Could you check a few things on this model? Use its own coordinates, in mm. Give positions to 0.01 mm unless a question says otherwise; leave off trailing zeros. Loops run counter-clockwise (first coordinate to the right, second up) from the corner with the lowest first, then second, coordinate; pieces in that order, holes last. Notation, with made-up numbers: M 34.5,79 L 82.5,79 A25 ccw 82.5,100 Z; hole C 38,-27.5 d10. An arc over 180 degrees is marked long. Return JSON: item names as keys, results as strings. Group by question number.
1. Please list where these lines run through material, in increasing order: line 1 (X direction, y = 13, z = -125); line 2 (Z direction, x = 20, y = 13); line 3 (X direction, y = 13.5, z = -129.5).
2. If we section it at B-B (y = 34.5): Write out the boundary of the cut face in (x, z), plus the area to 3 significant figures.
3. For pin 1 (0.5 mm diameter, centred on x = 0, z = 69.5, fed in from +Y); pin 2 (7 mm diameter, centred on x = -20.5, z = -127.5, fed in from +Y); pin 3 (4.5 mm diameter, centred on x = -19, z = -123, fed in from +Y), each with a flat end and sliding along its axis, tell me the tip position at first contact or that it passes through.
4. If we section it at C-C (x = 20.5): Write out the boundary of the cut face in (y, z).
5. If we section it at A-A (z = -125): Write out the boundary of the cut face in (x, y), plus the area to 3 significant figures.
6. If we section it at D-D (z = -32.5): Write out the boundary of the cut face in (x, y), plus the area to 3 significant figures.
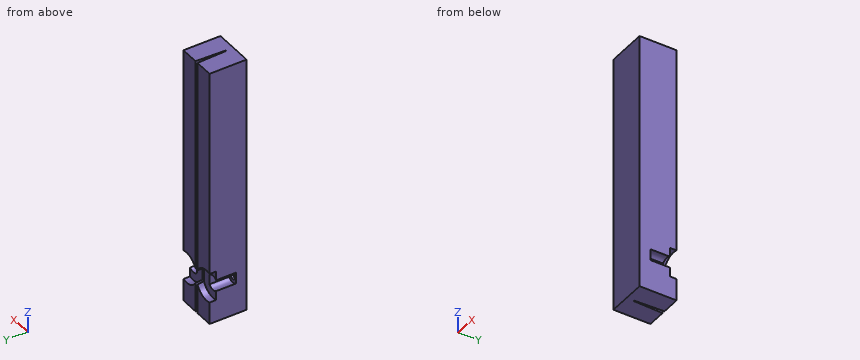
```python
from build123d import *

# Parameters (mm, degrees)
SKETCH1_W           = 54
SKETCH1_H           = 350
BOSS_EXTRUDE1_DEPTH = 50
CUT_EXTRUDE2_DEPTH  = 355.582853505
SKETCH7_R           = 21
SKETCH7_R_2         = 10
CUT_EXTRUDE4_DEPTH  = 9
CUT_EXTRUDE5_DEPTH  = 35.5
CUT_EXTRUDE6_DEPTH  = 3
CUT_EXTRUDE7_DEPTH  = 9


with BuildPart() as part:
    # Sketch1 → Boss-Extrude1 (new body)
    with BuildSketch(Plane(origin=(0, 0, 0), x_dir=(1, 0, 0), z_dir=(0, 1, 0))):
        Rectangle(SKETCH1_W, SKETCH1_H)
    extrude(amount=BOSS_EXTRUDE1_DEPTH)

    # Sketch3 → Cut-Extrude2 (cut, through all)
    with BuildSketch(Plane.XY.offset(175)):
        Polygon((-0.5, 10), (-2, 50), (2, 50), (0.5, 10), align=None)
    extrude(amount=-CUT_EXTRUDE2_DEPTH, mode=Mode.SUBTRACT)

    # Sketch7 → Cut-Extrude4 (cut)
    with BuildSketch(Plane(origin=(0, 50, 0), x_dir=(1, 0, 0), z_dir=(0, 1, 0))):
        with Locations((20.5, 125)):
            Circle(SKETCH7_R)
        with Locations((20.5, 125)):
            Circle(SKETCH7_R_2, mode=Mode.SUBTRACT)
    cut_extrude4 = extrude(amount=-CUT_EXTRUDE4_DEPTH, mode=Mode.SUBTRACT)

    # Sketch9 → Cut-Extrude5 (cut)
    with BuildSketch(Plane(origin=(0, 50, 0), x_dir=(1, 0, 0), z_dir=(0, 1, 0))):
        with BuildLine():
            Line((13, 131.614378278), (13, 118.385621722))
            ThreePointArc((13, 118.385621722), (30.5, 125), (13, 131.614378278))
        make_face()
    cut_extrude5 = extrude(amount=-CUT_EXTRUDE5_DEPTH, mode=Mode.SUBTRACT)

    # Sketch10 → Cut-Extrude6 (cut)
    with BuildSketch(Plane(origin=(0, 14.5, 0), x_dir=(1, 0, 0), z_dir=(0, 1, 0))):
        with BuildLine():
            Line((16.5, 128), (16.5, 122))
            ThreePointArc((16.5, 122), (25.5, 125), (16.5, 128))
        make_face()
    cut_extrude6 = extrude(amount=-CUT_EXTRUDE6_DEPTH, mode=Mode.SUBTRACT)

    # Sketch11 → Cut-Extrude7 (cut)
    with BuildSketch(Plane(origin=(0, 50, 0), x_dir=(1, 0, 0), z_dir=(0, 1, 0))):
        with BuildLine():
            Line((13, 131.614378278), (13, 118.385621722))
            ThreePointArc((13, 118.385621722), (10.5, 125), (13, 131.614378278))
        make_face()
    cut_extrude7 = extrude(amount=-CUT_EXTRUDE7_DEPTH, mode=Mode.SUBTRACT)

    # Mirror1: Cut-Extrude4, Cut-Extrude5, Cut-Extrude6, Cut-Extrude7 across plane
    add(cut_extrude4.mirror(Plane(origin=(0, 0, 0), x_dir=(0, 0, 1), z_dir=(1, 0, 0))), mode=Mode.SUBTRACT)
    add(cut_extrude5.mirror(Plane(origin=(0, 0, 0), x_dir=(0, 0, 1), z_dir=(1, 0, 0))), mode=Mode.SUBTRACT)
    add(cut_extrude6.mirror(Plane(origin=(0, 0, 0), x_dir=(0, 0, 1), z_dir=(1, 0, 0))), mode=Mode.SUBTRACT)
    add(cut_extrude7.mirror(Plane(origin=(0, 0, 0), x_dir=(0, 0, 1), z_dir=(1, 0, 0))), mode=Mode.SUBTRACT)


solid = part.part
```
Answer:
{
 "1": {"line 1": "x = -27 to -25.5, -16.5 to -0.61, 0.61 to 16.5, 25.5 to 27", "line 2": "z = -175 to -129.97, -120.03 to 175", "line 3": "x = -27 to -22.68, -18.32 to -0.63, 0.63 to 18.32, 22.68 to 27"},
 "2": {"outline": "M -27,-175 L -1.42,-175 L -1.42,175 L -27,175 L -27,-117.4 A10 cw -13,-118.39 L -13,-131.61 A10 cw -27,-132.6 Z; M 1.42,-175 L 27,-175 L 27,-132.6 A10 cw 13,-131.61 L 13,-118.39 A10 cw 27,-117.4 L 27,175 L 1.42,175 Z", "area": "17,400 mm²"},
 "3": {"pin 1": "stops at y = 10", "pin 2": "stops at y = 14.5", "pin 3": "stops at y = 11.5"},
 "4": {"outline": "M 0,-175 L 50,-175 L 50,-146 L 41,-146 L 41,-135 L 14.5,-135 L 14.5,-130 L 11.5,-130 L 11.5,-120 L 14.5,-120 L 14.5,-115 L 41,-115 L 41,-104 L 50,-104 L 50,175 L 0,175 Z"},
 "5": {"outline": "M -27,0 L 27,0 L 27,14.5 L 25.5,14.5 L 25.5,11.5 L 16.5,11.5 L 16.5,14.5 L 13,14.5 L 13,41 L 1.66,41 L 0.5,10 L -0.5,10 L -1.66,41 L -13,41 L -13,14.5 L -16.5,14.5 L -16.5,11.5 L -25.5,11.5 L -25.5,14.5 L -27,14.5 Z", "area": "1,350 mm²"},
 "6": {"outline": "M -27,0 L 27,0 L 27,50 L 2,50 L 0.5,10 L -0.5,10 L -2,50 L -27,50 Z", "area": "2,600 mm²"}
}
